Drawing for the job (mm, zero at the part's lowest x, y, z). Give positions to 0.01 mm unless a question says otherwise; leave off trailing zeros. Order: outer loops, then holes, each group sorted by start corner. A loop starts at its lowest first (then second) coordinate and runs counter-clockwise, first axis right, second up. Notation, with made-up numbers: (11, -39) - (46, -39) arc R30 cw to (46, 0) - close; hole circle Ø5 at (86.25, -15). An arc over 180 degrees is marked (long way). One line per item, written item: value.
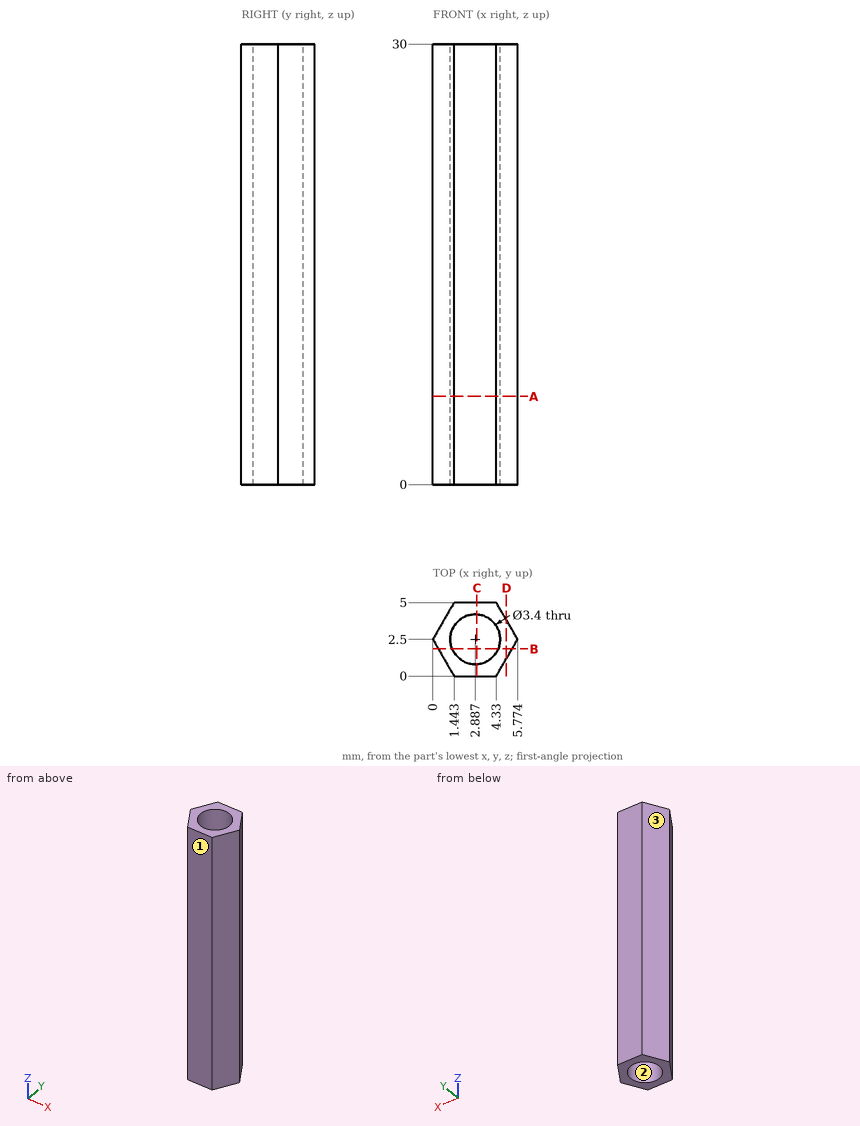
(1) Slice it at D-D, the plane x = 5. Give the cut face in (y, z).
Completed:
outline: (1.16, 0) - (3.84, 0) - (3.84, 30) - (1.16, 30) - close
(2) Pin check, flat tip, straight feed: P1, Ø3, axis at y = 2.5, z = 20, coming from the +X side. Stop position of the tip, or through.
Completed:
P1: x = 5.77
(3) Slice it at B-B, the plane y = 1.85. Give the cut face in (x, z) (1 decimal).
Completed:
outline: (0.4, 0) - (1.3, 0) - (1.3, 30) - (0.4, 30) - close; (4.5, 0) - (5.4, 0) - (5.4, 30) - (4.5, 30) - close
(4) Slice it at C-C, the plane x = 3. Give the cut face in (y, z).
Completed:
outline: (0, 0) - (0.8, 0) - (0.8, 30) - (0, 30) - close; (4.2, 0) - (5, 0) - (5, 30) - (4.2, 30) - close
(5) Pull direction Y, two halves, no side cores. Call the marked faces 1, 2 and 3: +Y half, -Y half, draft (parallel to the pull), parting line (faces both ways), or undercut.
Completed:
face 1: -Y half
face 2: undercut
face 3: +Y half
(6) Slice it at A-A, the plane z = 6. Give the cut face in (x, y).
Completed:
outline: (0, 2.5) - (1.44, 0) - (4.33, 0) - (5.77, 2.5) - (4.33, 5) - (1.44, 5) - close; hole circle Ø3.4 at (2.89, 2.5)
(7) Drill centre lines: line 1 (Y direction, x = 1.7, z = 8) (1 decimal); line 2 (Y direction, x = 4.15, z = 3.5) (1 decimal); line 3 (X direction, y = 1.4, z = 14.5) (1 decimal). Where is each one in solid material? Low to high.
Completed:
line 1: 0 to 1.3, 3.7 to 5
line 2: 0 to 1.4, 3.6 to 5
line 3: 0.6 to 1.6, 4.2 to 5.1
